from build123d import *


with BuildPart() as f1:
    # F0 (on Front) → F1 (revolve)
    with BuildSketch(Plane.XZ):
        with BuildLine():
            Line((36.743357, 2.401563), (36.743357, 8.751563))
            Line((36.743357, 8.751563), (4.993357, 8.751563))
            Line((4.993357, 8.751563), (4.993357, 7.481563))
            Line((4.993357, 7.481563), (3.723357, 7.481563))
            Line((3.723357, 7.481563), (3.723357, 8.751563))
            Line((3.723357, 8.751563), (-2.626643, 8.751563))
            Line((-2.626643, 8.751563), (-2.626643, 7.481563))
            Line((-2.626643, 7.481563), (-3.896643, 7.481563))
            Line((-3.896643, 7.481563), (-3.896643, 8.751563))
            Line((-3.896643, 8.751563), (-10.246643, 8.751563))
            Line((-10.246643, 8.751563), (-10.246643, 7.481563))
            Line((-10.246643, 7.481563), (-11.516643, 7.481563))
            Line((-11.516643, 7.481563), (-11.516643, 8.751563))
            Line((-11.516643, 8.751563), (-20.406643, 8.751563))
            Line((-20.406643, 8.751563), (-20.406643, 15.101563))
            ThreePointArc((-20.406643, 15.101563), (-23.581643, 18.276563), (-26.756643, 15.101563))
            Line((-26.756643, 15.101563), (-26.756643, 4.433563))
            Line((-26.756643, 4.433563), (-25.740643, 4.433563))
            Line((-25.740643, 4.433563), (-25.740643, 3.417563))
            Line((-25.740643, 3.417563), (-26.756643, 3.417563))
            Line((-26.756643, 3.417563), (-26.756643, 2.401563))
            Line((-26.756643, 2.401563), (36.743357, 2.401563))
        make_face()
    revolve(axis=Axis((36.743357, 0, 5.576563), (0, 0, -1)))


solid = f1.part
Verification items for the finished model (mm, model axes). A direction names the side the tool comes from. Round coordinates to 2 decimals unless told otherwise and drop trailing zeros. Answer in a Markdown table with one row per item. Add a question column.
Q1. Tool access check on faces 1 (the face through (38, 1, 2.402)), 2 (the face through (69.73, 1.45, 8.13)), 3 (the face through (83.5, -42, 3.418)). Record the directions out of +Z, -Z, +X, -X, +Y, -Y that give a thin tool (end or side, any length) a straight path to the whole face; none if there is none.
Q2. Release check for a two-part mould opening along Z. For faces 4 (the face through (76.075, 1.731, 8.108)), 5 (the face through (-5, -47, 4.434)), 6 (the face through (36, 0, 8.752)) record: pulls with the +Z half, pulls with the -Z half, needs draft (parallel to the pull), parting line crosses it, or undercut.
Q3. Gauge pin test, flat ends, axial feed: pin 1 (6 mm diameter, centred on y = 38.5, z = 4.5, fed in from +X); pin 2 (2 mm diameter, centred on y = 45.5, z = 10.5, fed in from +X); pin 3 (5 mm diameter, centred on x = 72.5, y = -0.5, fed in from +Z). Record the tip position at first contact, or that the pin passes through.
Q4. Material ranges on line 1 (X direction, y = 9, z = 17); line 2 (Z direction, x = -15.5, y = -12); line 3 (X direction, y = -34, z = 11.5), recorded low to high.
Found:
| question | item | result |
|---|---|---|
| 1 | face 1 | -Z, +X, -X, +Y, -Y |
| 1 | face 2 | +Z |
| 1 | face 3 | none |
| 2 | face 4 | needs draft |
| 2 | face 5 | undercut |
| 2 | face 6 | pulls with the +Z half |
| 3 | pin 1 | stops at x = 89.39 |
| 3 | pin 2 | stops at x = 82.04 |
| 3 | pin 3 | stops at z = 8.75 |
| 4 | line 1 | x = -25.48 to -20.33, 93.82 to 98.97 |
| 4 | line 2 | z = 2.4 to 8.75 |
| 4 | line 3 | x = -16.89 to -9.19, 82.68 to 90.37 |
